from build123d import *

# Parameters (mm, degrees)
F0_W     = 21.9
F0_H     = 4.9
F0_W_2   = 20.3
F0_H_2   = 3.3
F1_DEPTH = 30
F2_R     = 0.2
F3_R     = 1
F5_DEPTH = 0.8


with BuildPart() as f1:
    # F0 (on Top) → F1 (new body)
    with BuildSketch(Plane.XY):
        Rectangle(F0_W, F0_H)
        Rectangle(F0_W_2, F0_H_2, mode=Mode.SUBTRACT)
    extrude(amount=F1_DEPTH)

    # F2
    f2_edges = [f1.edges().sort_by_distance(p)[0] for p in [
        (-10.15, -1.65, 15),
        (10.15, 1.65, 15),
        (10.15, -1.65, 15),
        (-10.15, 1.65, 15),
    ]]
    fillet(f2_edges, radius=F2_R)

    # F3
    f3_edges = [f1.edges().sort_by_distance(p)[0] for p in [
        (10.95, -2.45, 15),
        (10.95, 2.45, 15),
        (-10.95, -2.45, 15),
        (-10.95, 2.45, 15),
    ]]
    fillet(f3_edges, radius=F3_R)

    # F4 (on face) → F5 (join)
    with BuildSketch(Plane(origin=(0, 0, 0), x_dir=(1, 0, 0), z_dir=(0, 0, -1))):
        with BuildLine():
            ThreePointArc((10.95, 1.45), (10.657107, 2.157107), (9.95, 2.45))
            Line((9.95, 2.45), (-9.95, 2.45))
            ThreePointArc((-9.95, 2.45), (-10.657107, 2.157107), (-10.95, 1.45))
            Line((-10.95, 1.45), (-10.95, -1.45))
            ThreePointArc((-10.95, -1.45), (-10.657107, -2.157107), (-9.95, -2.45))
            Line((-9.95, -2.45), (9.95, -2.45))
            ThreePointArc((9.95, -2.45), (10.657107, -2.157107), (10.95, -1.45))
            Line((10.95, -1.45), (10.95, 1.45))
        make_face()
    extrude(amount=F5_DEPTH)


solid = f1.part
Could you check a few things on this model? Use its own coordinates, in mm. A direction names the side the tool comes from. Give positions to 0.01 mm unless a question says otherwise; leave off trailing zeros. Order: outer loops, then holes, each group sorted by start corner. A loop starts at its lowest first (then second) coordinate and runs counter-clockwise, first axis right, second up. Notation, with made-up numbers: (64.25, 54) - (95.25, 54) arc R17 cw to (95.25, 59) - close; hole circle Ø5 at (44, 89.25). An arc over 180 degrees is marked (long way). Return JSON: item names as keys, results as strings. Group by question number.
Q1. Please list where these lines run through material, in increasing order: line 1 along Y through (x, z) = (9.25, 7); line 2 along X through (y, z) = (-0.4, 9). Write a range as [from, to].
Q2. Suppose I cut it at C-C, the plane y = 0.6. Please give me the cut outline in (x, z).
Q3. Which directions (+Z, -Z, +X, -X, +Y, -Y) give clear straight access to the entire face, cutting with the end or side of a thin tool? Please do faces 1 (the face through (-10.15, 0, 15)), 2 (the face through (0, 2.45, 15)).
Q4. Will this pin go through, and if not, where does the flat tip stop? pin 1 Ø1.5 at (x, y) = (4, -1.5) entering from +Z.
Q5. Thinking about a two-plate mould opening in X: for faces 3 (the face through (-10.95, 0, 15)), 4 (the face through (0, 1.65, 15)), 5 (the face through (10.95, 0, 15)), 6 (the face through (0, 2, 30)), which applies, pulls with the +X half, pulls with the -X half, needs draft (parallel to the pull), parting line crosses it, or undercut?
Q6. Suppose I cut it at B-B, the plane x = 8.75. Please give me the cut outline in (y, z).
Q7. Suppose I cut it at A-A, the plane z = 2.5. Please give me the cut outline in (x, y), and give its area (3 significant figures).
Resolved:
{
 "1": {"line 1": "y = [-2.45, -1.65], [1.65, 2.45]", "line 2": "x = [-10.95, -10.15], [10.15, 10.95]"},
 "2": {"outline": "(-10.95, -0.8) - (10.95, -0.8) - (10.95, 30) - (10.15, 30) - (10.15, 0) - (-10.15, 0) - (-10.15, 30) - (-10.95, 30) - close"},
 "3": {"face 1": "+Z", "face 2": "+Z, -Z, +X, -X, +Y"},
 "4": {"pin 1": "stops at z = 30"},
 "5": {"face 3": "pulls with the -X half", "face 4": "undercut", "face 5": "pulls with the +X half", "face 6": "needs draft"},
 "6": {"outline": "(-2.45, -0.8) - (2.45, -0.8) - (2.45, 30) - (1.65, 30) - (1.65, 0) - (-1.65, 0) - (-1.65, 30) - (-2.45, 30) - close"},
 "7": {"outline": "(-10.95, -1.45) arc R1 ccw to (-9.95, -2.45) - (9.95, -2.45) arc R1 ccw to (10.95, -1.45) - (10.95, 1.45) arc R1 ccw to (9.95, 2.45) - (-9.95, 2.45) arc R1 ccw to (-10.95, 1.45) - close; hole (-10.15, -1.45) arc R0.2 ccw to (-9.95, -1.65) - (9.95, -1.65) arc R0.2 ccw to (10.15, -1.45) - (10.15, 1.45) arc R0.2 ccw to (9.95, 1.65) - (-9.95, 1.65) arc R0.2 ccw to (-10.15, 1.45) - close", "area": "39.5 mm2"}
}
